from build123d import *

# Parameters (mm, degrees)
SKETCH_1_R      = 2
SKETCH_1_R_2    = 3
SKETCH_1_W      = 14.9
SKETCH_1_H      = 2.81
SKETCH_1_W_2    = 2.83
SKETCH_1_H_2    = 14.9
EXTRUDE_1_DEPTH = 6
FILLET_1_R      = 1
FILLET_2_R      = 5


with BuildPart() as part:
    # Эскиз1 → Бобышка-Вытянуть1 (new body)
    with BuildSketch(Plane(origin=(0, 0, 0), x_dir=(0, 0, -1), z_dir=(1, 0, 0))):
        Polygon((0, 0), (-20, 0), (-20, -215), (-40, -215), (-40, -235), (0, -235), align=None)
        with Locations((-16, -5)):
            Circle(SKETCH_1_R, mode=Mode.SUBTRACT)
        with Locations((-6, -5)):
            Circle(SKETCH_1_R, mode=Mode.SUBTRACT)
        with Locations((-11, -65)):
            Circle(SKETCH_1_R_2, mode=Mode.SUBTRACT)
        with Locations((-11, -180)):
            Circle(SKETCH_1_R_2, mode=Mode.SUBTRACT)
        with Locations((-20, -230.5)):
            Rectangle(SKETCH_1_W, SKETCH_1_H, mode=Mode.SUBTRACT)
        with Locations((-3.5, -95.5)):
            Rectangle(SKETCH_1_W_2, SKETCH_1_H_2, mode=Mode.SUBTRACT)
    extrude(amount=EXTRUDE_1_DEPTH)

    # Скругление1
    fillet_1_edges = [part.edges().sort_by_distance(p)[0] for p in [
        (3, -235, 40),
        (3, -215, 40),
        (3, 0, 20),
        (3, 0, 0),
    ]]
    fillet(fillet_1_edges, radius=FILLET_1_R)

    # Скругление2
    fillet_2_edges = [part.edges().sort_by_distance(p)[0] for p in [
        (3, -235, 0),
    ]]
    fillet(fillet_2_edges, radius=FILLET_2_R)


solid = part.part
CAD build for the part. Positions are in the model's coordinates, mm. A direction names the side the tool comes from. Round coordinates to 2 decimals unless told otherwise and drop trailing zeros. Order: outer loops, then holes, each group sorted by start corner. A loop starts at its lowest first (then second) coordinate and runs counter-clockwise, first axis right, second up. Notation, with made-up numbers: M 53.5,2 L 59.5,2 A20 ccw 59.5,36 Z; hole C 62,34 d6. An arc over 180 degrees is marked long. Use one line per item in the form item = value.
Q1. Saw through at B-B on x = 1.15. Give the cut face in (y, z) (3 decimals), then the cut area to 3 significant figures.
Recorded:
outline = M -235,5 A5 ccw -230,0 L -1,0 A1 ccw 0,1 L 0,19 A1 ccw -1,20 L -215,20 L -215,39 A1 ccw -216,40 L -234,40 A1 ccw -235,39 Z; hole M -231.905,12.55 L -229.095,12.55 L -229.095,27.45 L -231.905,27.45 Z; hole C -180,11 d6; hole M -102.95,2.085 L -88.05,2.085 L -88.05,4.915 L -102.95,4.915 Z; hole C -65,11 d6; hole C -5,6 d4; hole C -5,16 d4
area = 4,930 mm^2
Q2. Flat gauge pins, fed straight in: P1, Ø3, axis at x = 3, y = -97.5, coming from the +Z side; P2, Ø2.5, axis at x = 2.5, z = 3, coming from the -Y side; P3, Ø5, axis at y = -180, z = 11, coming from the -X side. Where does each tip first touch, or does it go through?
Recorded:
P1 = 20
P2 = -234.94
P3 = through
Q3. Which spindle directions (+Z, -Z, +X, -X, +Y, -Y) get a long thin tool onto all of the face, cutting with end or side? Do faces 4 (the flat face through (3, 0, 10)), 5 (the flat face through (3, -96, 4.915)). Say none if no direction does.
Recorded:
face_4 = +Z, -Z, +X, -X, +Y
face_5 = +X, -X
Q4. Saw through at D-D on y = -15.5. Give the cut face in (x, z).
Recorded:
outline = M 0,0 L 6,0 L 6,20 L 0,20 Z
Q5. Two-plate mould, pull along Z, no slides. Class faces 1 (the flat face through (3, -215, 29)), 2 (the flat face through (3, -107, 20)), 3 (the cylindrical face through (3, -6.2, 7.6)): +Z half, -Z half, draft (parallel to the pull), parting line (faces both ways), or undercut.
Recorded:
face_1 = draft
face_2 = +Z half
face_3 = undercut
Q6. Saw through at C-C on y = -180. Give the cut face in (x, z).
Recorded:
outline = M 0,0 L 6,0 L 6,8 L 0,8 Z; M 0,14 L 6,14 L 6,20 L 0,20 Z
Q7. Probe L1, parallel to Y at x = 4, z = 16 (3 decimals); L2, parallel to Y at x = 4.05, z = 11; L3, parallel to Z at x = 3, y = -91 (3 decimals). List the from-to ranges inside material, lowest first.
Recorded:
L1 = -235 to -231.905, -229.095 to -7, -3 to 0
L2 = -235 to -183, -177 to -68, -62 to 0
L3 = 0 to 2.085, 4.915 to 20
Q8. Saw through at A-A on z = 16. Give the cut face in (x, y) (3 decimals).
Recorded:
outline = M 0,-235 L 6,-235 L 6,-231.905 L 0,-231.905 Z; M 0,-229.095 L 6,-229.095 L 6,-7 L 0,-7 Z; M 0,-3 L 6,-3 L 6,0 L 0,0 Z
